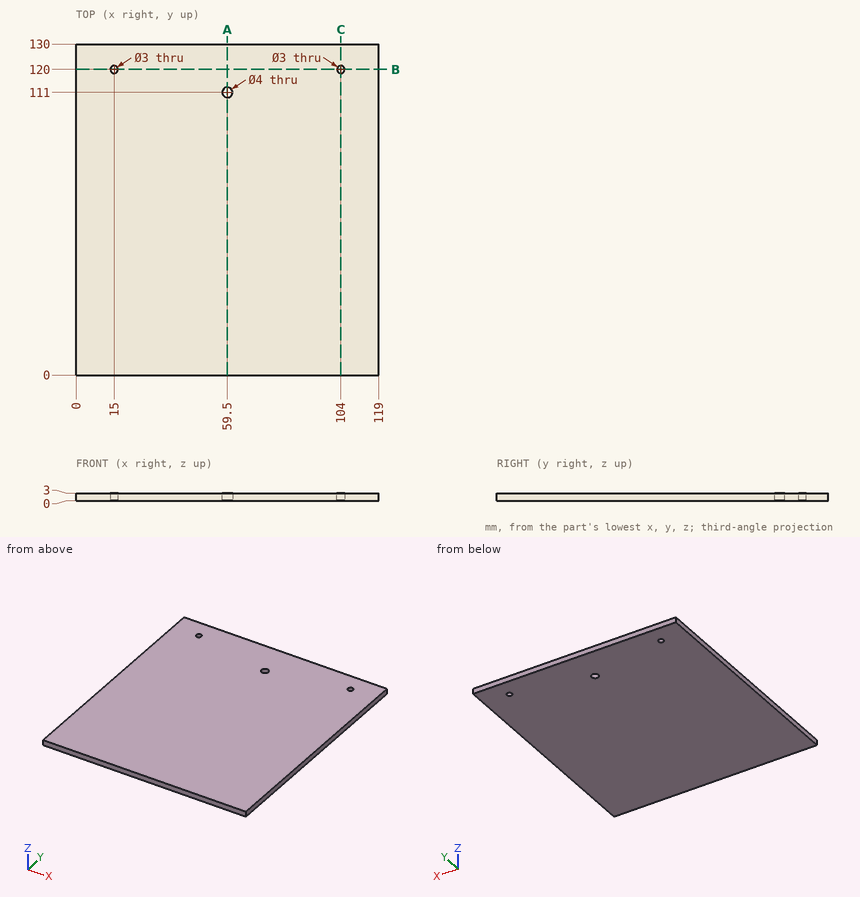
Check sheet for the drawn part. Datum: minimum x, y, z corner. Units: mm. Round coordinates to 2 decimals unless told otherwise and drop trailing zeros. Loops run counter-clockwise (first coordinate to the right, second up) from the corner with the lowest first, then second, coordinate; pieces in that order, holes last. Notation, with made-up numbers: M -8,62 L 5,62 A15 ccw 5,90 Z; hole C -34.5,1 d7. An arc over 180 degrees is marked long. One line per question, with ' | ' between items. Start each with the question number.
Item 1: Section check B-B (y = 120). Record the boundary of the cut face in (x, z), and give its area (3 significant figures).
Item 2: Section check C-C (x = 104). Record the boundary of the cut face in (y, z).
Item 3: Section check A-A (x = 59.5). Record the boundary of the cut face in (y, z).
Item 4: Scan lines: probe 1 along X at (y, z) = (120, 1.35); probe 2 along Y at (x, z) = (15, 0.7); probe 3 along Y at (x, z) = (60, 0.8). Record each from-to range of solid material in increasing order.
Worked out:
1) outline: M 0,0 L 13.5,0 L 13.5,3 L 0,3 Z; M 16.5,0 L 102.5,0 L 102.5,3 L 16.5,3 Z; M 105.5,0 L 119,0 L 119,3 L 105.5,3 Z | area: 339 mm^2
2) outline: M 0,0 L 118.5,0 L 118.5,3 L 0,3 Z; M 121.5,0 L 130,0 L 130,3 L 121.5,3 Z
3) outline: M 0,0 L 109,0 L 109,3 L 0,3 Z; M 113,0 L 130,0 L 130,3 L 113,3 Z
4) probe 1: 0 to 13.5, 16.5 to 102.5, 105.5 to 119 | probe 2: 0 to 118.5, 121.5 to 130 | probe 3: 0 to 109.06, 112.94 to 130
